Check sheet for the modelled part. Datum: model origin and axes. Units: mm. A direction names the side the tool comes from. Give positions to 0.01 mm unless a question says otherwise; leave off trailing zeros. Write each loop counter-clockwise with the first axis right and the second up, starting at its lowest first coordinate (ties: lowest second). Pieces come first, ordered by that corner, then holes.
from build123d import *

# Parameters (mm, degrees)
F0_W      = 12.7
F0_H      = 1219.2
F1_DEPTH  = 25.4
F2_W      = 406.4
F2_H      = 1396.9661742449
F2_W_2    = 69.85
F2_H_2    = 1270
F2_W_3    = 63.5
F3_DEPTH  = 25.4
F4_W      = 25.4
F4_H      = 1270
F5_DEPTH  = 25.4
F6_W      = 25.4
F6_H      = 1270
F7_DEPTH  = 25.4
F6_H_2    = 25.4
F6_W_2    = 31.75
F6_H_3    = 1244.6
F9_W      = 975.7457971573
F9_H      = 1423.7642139196
F10_DEPTH = 218.67692


with BuildPart() as f1:
    # F0 (on Front) → F1 (new body)
    with BuildSketch(Plane.XZ):
        Polygon((-930.275, 1270), (-930.275, 1244.6), (-771.525, 1244.6), (-758.825, 1244.6), (-631.825, 1244.6), (-619.125, 1244.6), (-492.125, 1244.6), (-479.425, 1244.6), (-352.425, 1244.6), (-339.725, 1244.6), (-212.725, 1244.6), (-200.025, 1244.6), (-73.025, 1244.6), (-60.325, 1244.6), (66.675, 1244.6), (79.375, 1244.6), (206.375, 1244.6), (219.075, 1244.6), (346.075, 1244.6), (358.775, 1244.6), (485.775, 1244.6), (498.475, 1244.6), (625.475, 1244.6), (638.175, 1244.6), (765.175, 1244.6), (777.875, 1244.6), (930.275, 1244.6), (930.275, 1270), align=None)
        with Locations((-765.175, 635)):
            Rectangle(F0_W, F0_H)
        Polygon((-758.825, 25.4), (-771.525, 25.4), (-930.275, 25.4), (-930.275, 0), (930.275, 0), (930.275, 25.4), (777.875, 25.4), (765.175, 25.4), (638.175, 25.4), (625.475, 25.4), (498.475, 25.4), (485.775, 25.4), (358.775, 25.4), (346.075, 25.4), (219.075, 25.4), (206.375, 25.4), (79.375, 25.4), (66.675, 25.4), (-60.325, 25.4), (-73.025, 25.4), (-200.025, 25.4), (-212.725, 25.4), (-339.725, 25.4), (-352.425, 25.4), (-479.425, 25.4), (-492.125, 25.4), (-619.125, 25.4), (-631.825, 25.4), align=None)
        with Locations((771.525, 635)):
            Rectangle(F0_W, F0_H)
        with Locations((-625.475, 635)):
            Rectangle(F0_W, F0_H)
        with Locations((-485.775, 635)):
            Rectangle(F0_W, F0_H)
        with Locations((-346.075, 635)):
            Rectangle(F0_W, F0_H)
        with Locations((-206.375, 635)):
            Rectangle(F0_W, F0_H)
        with Locations((-66.675, 635)):
            Rectangle(F0_W, F0_H)
        with Locations((73.025, 635)):
            Rectangle(F0_W, F0_H)
        with Locations((212.725, 635)):
            Rectangle(F0_W, F0_H)
        with Locations((352.425, 635)):
            Rectangle(F0_W, F0_H)
        with Locations((492.125, 635)):
            Rectangle(F0_W, F0_H)
        with Locations((631.825, 635)):
            Rectangle(F0_W, F0_H)
    extrude(amount=F1_DEPTH)

    # F2 (on face) → F3 (cut)
    with BuildSketch(Plane.XZ.offset(25.4)):
        with Locations((3.175, 593.5398563743)):
            Rectangle(F2_W, F2_H)
        with Locations((-895.35, 635)):
            Rectangle(F2_W_2, F2_H_2)
        with Locations((898.525, 635)):
            Rectangle(F2_W_3, F2_H_2)
    extrude(amount=-F3_DEPTH, mode=Mode.SUBTRACT)

    # F4 (on face) → F5, piece 2 (join)
    with BuildSketch(Plane.XZ.offset(25.4)):
        with Locations((879.475, 635)):
            Rectangle(F4_W, F4_H)
    extrude(amount=-F5_DEPTH)

    # F6 (on face) → F7, piece 2 (join)
    with BuildSketch(Plane.XZ.offset(25.4)):
        with Locations((911.225, 1257.3)):
            Rectangle(F6_W, F6_H_2)
        with Locations((882.65, 1257.3)):
            Rectangle(F6_W_2, F6_H_2)
        with Locations((911.225, 622.3)):
            Rectangle(F6_W, F6_H_3)
    extrude(amount=-F7_DEPTH)

    # F8: union 


with BuildPart() as f5:
    # F4 (on face) → F5 (new body)
    with BuildSketch(Plane.XZ.offset(25.4)):
        with Locations((-873.125, 635)):
            Rectangle(F4_W, F4_H)
    extrude(amount=-F5_DEPTH)


with BuildPart() as f7:
    # F6 (on face) → F7 (new body)
    with BuildSketch(Plane.XZ.offset(25.4)):
        with Locations((-904.875, 635)):
            Rectangle(F6_W, F6_H)
    extrude(amount=-F7_DEPTH)


with BuildPart() as f10_tool:
    # F9 (on face) → F10 (new body)
    with BuildSketch(Plane(origin=(0, 0, 0), x_dir=(-1, 0, 0), z_dir=(0, 1, 0))):
        with Locations((666.6726469994, 601.2135818601)):
            Rectangle(F9_W, F9_H)
    extrude(amount=-F10_DEPTH)


with BuildPart() as f1_1:
    add(f1.part)

    # F10: cut by f10_tool
    add(f10_tool.part, mode=Mode.SUBTRACT)


with BuildPart() as f5_1:
    add(f5.part)

    # F10: cut by f10_tool
    add(f10_tool.part, mode=Mode.SUBTRACT)


with BuildPart() as f7_1:
    add(f7.part)

    # F10: cut by f10_tool
    add(f10_tool.part, mode=Mode.SUBTRACT)


solid = f1_1.part
1) Gauge pin test, flat ends, axial feed: pin 1 (6 mm diameter, centred on x = 735.5, y = -14.5, fed in from -Z); pin 2 (1.9 mm diameter, centred on x = 895, y = -9.5, fed in from -Z). Record the tip position at first contact, or that the pin passes through.
2) Draft check along Z on faces 1 (the flat face through (822, -13, 1244.6)), 2 (the flat face through (892.175, -13, 614)), 3 (the flat face through (544, -13, 0)). Enter one of: +Z half, -Z half, draft (parallel to the pull), parting line (faces both ways), or undercut.
3) Sectioned sample at A-A on z = 1168. Record the boundary of the cut face in (x, y) (3 decimals).
4) Sectioned sample at C-C on x = 263. Record the boundary of the cut face in (y, z), then the cut area to 3 significant figures.
5) Scan line: L1, parallel to Z at x = 830.5, y = -6.75. Record every from-to range of solid material in increasing order.
6) Access from +Z, -Z, +X, -X, +Y, -Y to the whole of each face (thin tool, end or side, straight path). Record for faces 4 (the flat face through (570, -13, 1270)), 5 (the flat face through (358.775, -13, 626)).
7) Sectioned sample at B-B on y = -15.5. Record the boundary of the cut face in (x, z) (3 decimals), then the cut area to 3 significant figures.
Answers below:
1. pin 1: stops at z = 0
1. pin 2: stops at z = 1244.6
2. face 1: undercut
2. face 2: draft
2. face 3: -Z half
3. outline: (206.375, -25.4) - (219.075, -25.4) - (219.075, 0) - (206.375, 0) - close; (346.075, -25.4) - (358.775, -25.4) - (358.775, 0) - (346.075, 0) - close; (485.775, -25.4) - (498.475, -25.4) - (498.475, 0) - (485.775, 0) - close; (625.475, -25.4) - (638.175, -25.4) - (638.175, 0) - (625.475, 0) - close; (765.175, -25.4) - (777.875, -25.4) - (777.875, 0) - (765.175, 0) - close; (866.775, -25.4) - (892.175, -25.4) - (892.175, 0) - (866.775, 0) - close; (898.525, -25.4) - (923.925, -25.4) - (923.925, 0) - (898.525, 0) - close
4. outline: (-25.4, 0) - (0, 0) - (0, 25.4) - (-25.4, 25.4) - close; (-25.4, 1244.6) - (0, 1244.6) - (0, 1270) - (-25.4, 1270) - close
4. area: 1,290 mm2
5. L1: z = 0 to 25.4, 1244.6 to 1270
6. face 4: +Z, +X, -X, +Y, -Y
6. face 5: +Y, -Y
7. outline: (206.375, 0) - (892.175, 0) - (892.175, 1244.6) - (898.525, 1244.6) - (898.525, 0) - (923.925, 0) - (923.925, 1270) - (206.375, 1270) - close; hole (219.075, 25.4) - (346.075, 25.4) - (346.075, 1244.6) - (219.075, 1244.6) - close; hole (358.775, 25.4) - (485.775, 25.4) - (485.775, 1244.6) - (358.775, 1244.6) - close; hole (498.475, 25.4) - (625.475, 25.4) - (625.475, 1244.6) - (498.475, 1244.6) - close; hole (638.175, 25.4) - (765.175, 25.4) - (765.175, 1244.6) - (638.175, 1244.6) - close; hole (777.875, 25.4) - (866.775, 25.4) - (866.775, 1244.6) - (777.875, 1244.6) - close
7. area: 176,000 mm2
